Part model, mm, in its own coordinate system. A direction names the side the tool comes from. Coordinates: 2 decimals unless noted, no trailing zeros. Loops run counter-clockwise (first coordinate to the right, second up) from the corner with the lowest first, then second, coordinate; pieces in that order, holes last. Notation, with made-up numbers: (-15, 82) - (14, 82) arc R17 ccw to (14, 91) - close; hole circle Ø9 at (-11, 52). An arc over 180 degrees is marked (long way). Use a Markdown table: item, result. Add a question column.
1. Band-saw the part on B-B, the plane x = -5. Give the cut face in (y, z), plus the area to 3 significant figures.
2. Band-saw the part on C-C, the plane y = 10. Give the cut face in (x, z).
3. Drop flat-ended pins along their axis: pin 1 (2 mm diameter, centred on x = 5, y = 17, fed in from +Z); pin 2 (1 mm diameter, centred on y = 18.5, z = 1, fed in from +X); pin 3 (2 mm diameter, centred on x = 4.5, z = -3.5, fed in from -Y); pin 4 (1.5 mm diameter, centred on x = -1.5, y = 13.5, fed in from -Z). Give the stop position or say it passes through.
4. Band-saw the part on D-D, the plane y = 20.25. Give the cut face in (x, z).
5. 3-axis set-ups, long thin cutter, end or side, ignore diameter. For faces 1 (the cylindrical face through (-4.724, 12.135, 3.622)), 2 (the flat face through (-8.349, 2.317, 4.586)): which of +Z, -Z, +X, -X, +Y, -Y reach the whole face in a straight line?
6. Wall check: probe 1 along Y at (x, z) = (-8, 4.75); probe 2 along Y at (x, z) = (-2, -1.5); probe 3 along Z at (x, y) = (3.25, 5.5). Give the ranges that are in metal, low to high. Write a range as [from, to].
7. Band-saw the part on A-A, the plane y = 3. Give the cut face in (x, z).
from build123d import *

# Parameters (mm, degrees)
BOSS_EXTRUDE1_DEPTH = 4.7
SKETCH2_R           = 5.953125
BOSS_EXTRUDE2_DEPTH = 15.08125


with BuildPart() as part:
    # Sketch1 → Boss-Extrude1 (new body)
    with BuildSketch(Plane(origin=(0, 0, 0), x_dir=(1, 0, 0), z_dir=(0, 1, 0))):
        Polygon((5.624451566, 9.451615977), (-5.37311376, 9.596725927), (-10.997565326, 0.14510995), (-5.624451566, -9.451615977), (5.37311376, -9.596725927), (10.997565326, -0.14510995), align=None)
    extrude(amount=BOSS_EXTRUDE1_DEPTH)

    # Sketch2 → Boss-Extrude2 (add)
    with BuildSketch(Plane(origin=(0, 4.7, 0), x_dir=(1, 0, 0), z_dir=(0, 1, 0))):
        Circle(SKETCH2_R)
    extrude(amount=BOSS_EXTRUDE2_DEPTH)

    # Sketch4 → Revolve1 (revolve)
    with BuildSketch(Plane(origin=(0, 0, 0), x_dir=(0, 0, -1), z_dir=(1, 0, 0))):
        Polygon((0, 19.78125), (0, 23.75), (3.96875, 19.78125), align=None)
    revolve(axis=Axis((0, 19.78125, 0), (0, 1, 0)))


solid = part.part
Geometry check:
| question | item | result |
|---|---|---|
| 1 | outline | (0, -9.59) - (4.7, -9.59) - (4.7, -3.23) - (19.78, -3.23) - (19.78, 3.23) - (4.7, 3.23) - (4.7, 9.46) - (0, 9.46) - close |
| 1 | area | 187 mm^2 |
| 2 | outline | circle Ø11.91 at (0, 0) |
| 3 | pin 1 | stops at z = 4.41 |
| 3 | pin 2 | stops at x = 5.93 |
| 3 | pin 3 | stops at y = 0 |
| 3 | pin 4 | stops at z = -5.91 |
| 4 | outline | circle Ø7 at (0, 0) |
| 5 | face 1 | +Y |
| 5 | face 2 | +Z, -X, +Y, -Y |
| 6 | probe 1 | y = [0, 4.7] |
| 6 | probe 2 | y = [0, 21.25] |
| 6 | probe 3 | z = [-4.99, 4.99] |
| 7 | outline | (-11, -0.15) - (-5.37, -9.6) - (5.62, -9.45) - (11, 0.15) - (5.37, 9.6) - (-5.62, 9.45) - close |
